Read the model definition and answer for the solid it produces. Units are mm, in the model's axes. Face numbers are marked on the shaded views. A direction names the side the tool comes from. Give positions to 0.01 mm unless a question says otherwise; leave off trailing zeros. Order: outer loops, then holes, each group sorted by start corner. A loop starts at its lowest first (then second) coordinate and runs counter-clockwise, first axis right, second up. Notation, with made-up numbers: (8.5, -33.5) - (50.5, -33.5) arc R15 ccw to (50.5, -5.5) - close; hole circle Ø1 at (48, 66). An arc over 180 degrees is marked (long way). Write each question's results on one line, items separated by ' | '. Start each with the question number.
Q1. Find section A-A on z = -34. Give the vertices of the cut face in (x, y).
Q2. Flat-ended cylindrical pins translate along their axes: P1, Ø15.5, axis at x = 25, y = -22, coming from the +Z side; P2, Ø8.5, axis at y = -19.05, z = -10, coming from the +X side; P3, Ø5, axis at y = -13.5, z = -51, coming from the -X side. Find the tip coordinate at first contact, or state that the pin passes through.
Q3. For a pull along X with two mould halves and no side action, classify the marked faces 4, 5, 6 and 7 as +X half, -X half, draft (parallel to the pull), parting line (faces both ways), or undercut.
Q4. Find the intervals of material crossed by line 1 along Z through (x, y) = (32, -19); line 2 along X through (y, z) = (1.75, -66); line 3 along X through (y, z) = (-28, -87.5), in increasing order. Write a range as from..to.
Q5. A tool of negligible diameter and unlimited length cuts with its end or side. For the marked faces 1, 2 and 3, from which of +Z, -Z, +X, -X, +Y, -Y can it reach the whole face along a straight path? Write none if from no direction.
Q6. Find section B-B on y = -26.5. Give the vertices of the cut face in (x, z).
Q7. Find section C-C on x = 92.5. Give the vertices of the cut face in (y, z).
Q8. Find section D-D on z = -10. Give the vertices of the cut face in (x, y), and give its area (3 significant figures).
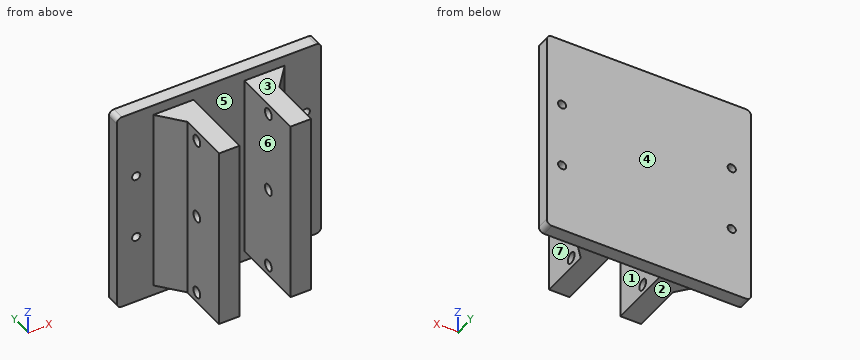
from build123d import *

# Parameters (mm, degrees)
SKETCH1_R           = 2
BOSS_EXTRUDE1_DEPTH = 6.35
SKETCH4_W           = 10
SKETCH4_H           = 90
BOSS_EXTRUDE2_DEPTH = 36.75
SKETCH5_R           = 2.7
CUT_EXTRUDE1_DEPTH  = 129.867422183
BOSS_EXTRUDE3_DEPTH = 90


with BuildPart() as part:
    # Sketch1 → Boss-Extrude1 (new body)
    with BuildSketch(Plane(origin=(0, 0, 0), x_dir=(1, 0, 0), z_dir=(0, 1, 0))):
        with BuildLine():
            Line((2.5, 0), (97.5, 0))
            ThreePointArc((97.5, 0), (99.267766953, 0.732233047), (100, 2.5))
            Line((100, 2.5), (100, 97.5))
            ThreePointArc((100, 97.5), (99.267766953, 99.267766953), (97.5, 100))
            Line((97.5, 100), (2.5, 100))
            ThreePointArc((2.5, 100), (0.732233047, 99.267766953), (0, 97.5))
            Line((0, 97.5), (0, 2.5))
            ThreePointArc((0, 2.5), (0.732233047, 0.732233047), (2.5, 0))
        make_face()
        with Locations(Location((9.5, 34, 0), (0, 0, 270))):
            Circle(SKETCH1_R, mode=Mode.SUBTRACT)
        with Locations(Location((9.5, 66, 0), (0, 0, 270))):
            Circle(SKETCH1_R, mode=Mode.SUBTRACT)
        with Locations(Location((92.5, 66, 0), (0, 0, 270))):
            Circle(SKETCH1_R, mode=Mode.SUBTRACT)
        with Locations(Location((92.5, 34, 0), (0, 0, 270))):
            Circle(SKETCH1_R, mode=Mode.SUBTRACT)
    extrude(amount=BOSS_EXTRUDE1_DEPTH)

    # Sketch4 → Boss-Extrude2 (add)
    with BuildSketch(Plane(origin=(0, 0, 0), x_dir=(1, 0, 0), z_dir=(0, 1, 0))):
        with Locations((32.5, 50)):
            Rectangle(SKETCH4_W, SKETCH4_H)
        with Locations((67.5, 50)):
            Rectangle(SKETCH4_W, SKETCH4_H)
    extrude(amount=-BOSS_EXTRUDE2_DEPTH)

    # Sketch5 → Cut-Extrude1 (cut, through all)
    with BuildSketch(Plane.ZY.offset(-27.5)):
        with Locations((-90, -19.05)):
            Circle(SKETCH5_R)
        with Locations((-50, -19.05)):
            Circle(SKETCH5_R)
        with Locations((-10, -19.05)):
            Circle(SKETCH5_R)
    extrude(amount=-CUT_EXTRUDE1_DEPTH, mode=Mode.SUBTRACT)

    # Sketch6 → Boss-Extrude3 (add)
    with BuildSketch(Plane.XY.offset(-5)):
        Polygon((72.5, 0), (82.141814145, 0), (72.5, -11.490666647), align=None)
        Polygon((27.5, 0), (17.858185855, 0), (27.5, -11.490666647), align=None)
    extrude(amount=-BOSS_EXTRUDE3_DEPTH)


solid = part.part
Working result:
1) outline: (0, 0) - (7.5, 0) - (7.5, 6.35) - (0, 6.35) - close; (11.5, 0) - (17.86, 0) - (27.5, -11.49) - (27.5, -36.75) - (37.5, -36.75) - (37.5, 0) - (62.5, 0) - (62.5, -36.75) - (72.5, -36.75) - (72.5, -11.49) - (82.14, 0) - (90.5, 0) - (90.5, 6.35) - (11.5, 6.35) - close; (94.5, 0) - (100, 0) - (100, 6.35) - (94.5, 6.35) - close
2) P1: z = -5 | P2: x = 72.5 | P3: x = 27.09
3) face 4: draft | face 5: undercut | face 6: undercut | face 7: +X half
4) line 1: -95..-92.7, -87.3..-52.7, -47.3..-12.7, -7.3..-5 | line 2: 0..7.5, 11.5..90.5, 94.5..100 | line 3: 27.5..37.5, 62.5..72.5
5) face 1: +Z, -Z, -Y | face 2: -Z, +X, -X, -Y | face 3: +Z, +X, -X, -Y
6) outline: (27.5, -95) - (37.5, -95) - (37.5, -5) - (27.5, -5) - close; (62.5, -95) - (72.5, -95) - (72.5, -5) - (62.5, -5) - close
7) outline: (0, -100) - (6.35, -100) - (6.35, -68) - (0, -68) - close; (0, -64) - (6.35, -64) - (6.35, -36) - (0, -36) - close; (0, -32) - (6.35, -32) - (6.35, 0) - (0, 0) - close
8) outline: (0, 0) - (17.86, 0) - (27.5, -11.49) - (27.5, -16.35) - (37.5, -16.35) - (37.5, 0) - (62.5, 0) - (62.5, -16.35) - (72.5, -16.35) - (72.5, -11.49) - (82.14, 0) - (100, 0) - (100, 6.35) - (0, 6.35) - close; (27.5, -36.75) - (37.5, -36.75) - (37.5, -21.75) - (27.5, -21.75) - close; (62.5, -36.75) - (72.5, -36.75) - (72.5, -21.75) - (62.5, -21.75) - close | area: 1,370 mm²
